from build123d import *

# Parameters (mm, degrees)
ESQUISSE1_W             = 5
ESQUISSE1_H             = 30
BOSS_EXTRU_1_DEPTH      = 35
ENL_V_MAT_EXTRU_1_DEPTH = 39.405728739
ESQUISSE3_R             = 1.5
ESQUISSE3_R_2           = 2
ENL_V_MAT_EXTRU_2_DEPTH = 40
ESQUISSE4_W             = 2.5
ESQUISSE4_H             = 7
ENL_V_MAT_EXTRU_3_DEPTH = 10


with BuildPart() as part:
    # Esquisse1 → Boss.-Extru.1 (new body)
    with BuildSketch(Plane.XY):
        Rectangle(ESQUISSE1_W, ESQUISSE1_H)
    extrude(amount=BOSS_EXTRU_1_DEPTH)

    # Esquisse2 → Enlèv. mat.-Extru.1 (cut, through all)
    with BuildSketch(Plane(origin=(2.5, 0, 0), x_dir=(0, 0, -1), z_dir=(1, 0, 0))):
        with BuildLine():
            Line((-10, -2), (-25, -2))
            ThreePointArc((-25, -2), (-27, 0), (-25, 2))
            Line((-25, 2), (-10, 2))
            ThreePointArc((-10, 2), (-8, 0), (-10, -2))
        make_face()
    extrude(amount=-ENL_V_MAT_EXTRU_1_DEPTH, mode=Mode.SUBTRACT)

    # Esquisse3 → Enlèv. mat.-Extru.2 (cut)
    with BuildSketch(Plane.XY.offset(35)):
        Circle(ESQUISSE3_R)
        with Locations((0, -12)):
            Circle(ESQUISSE3_R_2)
        with Locations(Location((0, 12, 0), (0, 0, 180))):
            Circle(ESQUISSE3_R_2)
    extrude(amount=-ENL_V_MAT_EXTRU_2_DEPTH, mode=Mode.SUBTRACT)

    # Esquisse4 → Enlèv. mat.-Extru.3 (cut)
    with BuildSketch(Plane(origin=(2.5, 0, 0), x_dir=(0, 0, -1), z_dir=(1, 0, 0))):
        with Locations((-31, 0)):
            Rectangle(ESQUISSE4_W, ESQUISSE4_H)
    enl_v_mat_extru_3 = extrude(amount=-ENL_V_MAT_EXTRU_3_DEPTH, mode=Mode.SUBTRACT)

    # Symétrie1: Enlèv. mat.-Extru.3 across plane
    add(enl_v_mat_extru_3.mirror(Plane.XY.offset(17.5)), mode=Mode.SUBTRACT)


solid = part.part
Geometry: final body of the model. Coordinates: model frame, mm. A direction names the side the tool comes from. Give positions to 0.01 mm unless a question says otherwise; leave off trailing zeros. Write each loop counter-clockwise with the first axis right and the second up, starting at its lowest first coordinate (ties: lowest second). Pieces come first, ordered by that corner, then holes. Notation, with made-up numbers: (-33, 29.5) -> (12, 29.5) arc R13 ccw to (12, 39.5) -> close; hole circle Ø7 at (22, 25.25). An arc over 180 degrees is marked (long way). Answer as a JSON object with one key per item and string values.
1. Cut plane C-C on y = 0. Count the separate pieces of the cut face and the enclosed holes in it, and give its area (3 significant figures).
Ans:
{"separate pieces": "8", "enclosed holes": "0", "area": "22.0 mm^2"}
2. Ray query, probe 1 along Z at (x, y) = (-0.25, 2.5); probe 2 along Y at (x, z) = (0, 1.5); probe 3 along Y at (x, z) = (0, 30). Return the intervals inside material, ascending. Write a range as from..to.
Ans:
{"probe 1": "z = 0..2.75, 5.25..29.75, 32.25..35", "probe 2": "y = -15..-14, -10..-1.5, 1.5..10, 14..15", "probe 3": "y = -15..-14, -10..-3.5, 3.5..10, 14..15"}
3. Mould query, pull axis Y, two halves, no side actions, for faces 3 (the flat face through (0, 2, 29.75)), 4 (the cylindrical face through (-1.5, 0.07, 33.64)), 5 (the flat face through (2.5, -4, 17)), 6 (the flat face through (0, -15, 17)). Classes: pulls with the +Y half, pulls with the -Y half, needs draft (parallel to the pull), parting line crosses it, or undercut.
Ans:
{"face 3": "undercut", "face 4": "undercut", "face 5": "needs draft", "face 6": "pulls with the -Y half"}
4. Cut plane D-D on z = 7.5. Output: boundary loops of the cut face in (x, y).
Ans:
{"outline": "(-2.5, -15) -> (2.5, -15) -> (2.5, 15) -> (-2.5, 15) -> close; hole circle Ø4 at (0, -12); hole circle Ø4 at (0, 12); hole circle Ø3 at (0, 0)"}
5. Access query for faces 1 (the flat face through (0, -3.5, 4)), 2 (the cylindrical face through (-1.5, 0.07, 6.61)). Directions: +Z, -Z, +X, -X, +Y, -Y. A direction counts if a zero-diameter tool reaches every point of the face in a straight line with its end or side. Return the directions, or none.
Ans:
{"face 1": "+X, -X", "face 2": "+Z, -Z"}
6. Cut plane B-B on y = -12. Output: boundary loops of the cut face in (x, z).
Ans:
{"outline": "(-2.5, 0) -> (-2, 0) -> (-2, 35) -> (-2.5, 35) -> close; (2, 0) -> (2.5, 0) -> (2.5, 35) -> (2, 35) -> close"}
7. Cut plane A-A on z = 16.5. Output: boundary loops of the cut face in (x, y), and give its area (3 significant figures).
Ans:
{"outline": "(-2.5, -15) -> (2.5, -15) -> (2.5, -2) -> (-2.5, -2) -> close; (-2.5, 2) -> (2.5, 2) -> (2.5, 15) -> (-2.5, 15) -> close; hole circle Ø4 at (0, -12); hole circle Ø4 at (0, 12)", "area": "105 mm^2"}
